CAD build for the part. Positions are in the model's coordinates, mm. A direction names the side the tool comes from. Give positions to 0.01 mm unless a question says otherwise; leave off trailing zeros. Write each loop counter-clockwise with the first axis right and the second up, starting at its lowest first coordinate (ties: lowest second). Pieces come first, ordered by that corner, then holes. Notation, with made-up numbers: M 48,37.25 L 81,37.25 A23 ccw 81,58.25 Z; hole C 31.25,49.25 d3. An arc over 180 degrees is marked long. One line per question, with ' | ' between items. Start each with the question number.
1. Cut at D-D, the plane x = 46.5. Write the cut outline in (y, z).
2. Wall check: L1, parallel to Y at x = -17.67, z = 1.6; L2, parallel to X at y = 0.75, z = 1.4; L3, parallel to X at y = -4, z = 0.7. Give the ranges that are in metal, low to high.
3. Cut at A-A, the plane y = 0. Write the cut outline in (x, z), then the cut area to 3 significant figures.
4. Pull direction Y, two halves, no side cores. Call faces 3 (the face through (18, 1, 0)), 4 (the face through (50.036, -2.721, 0.986)), 5 (the face through (-19.42, 0.08, 0.99)), 6 (the face through (1.617, -0.67, 0.986)): released by +Y, released by -Y, zero draft, split by the parting line, or undercut.
5. Cut at C-C, the plane z = 1.1. Write the cut outline in (x, y) (3 decimals), then the cut area to 3 significant figures.
6. Which spindle directions (+Z, -Z, +X, -X, +Y, -Y) get a long thin tool onto all of the face, cutting with end or side? Do faces 1 (the face through (-14.26, 4.01, 0.99)), 2 (the face through (-10, -3.125, 1)). Say none if no direction does.
7. Cut at B-B, the plane x = -17.67. Write the cut outline in (y, z), then the cut area to 3 significant figures.
```python
from build123d import *

# Parameters (mm, degrees)
SKETCH1_R           = 1.75
BOSS_EXTRUDE1_DEPTH = 2


with BuildPart() as part:
    # Sketch1 → Boss-Extrude1 (new body)
    with BuildSketch(Plane.XY):
        with BuildLine():
            Line((-1.959177489, 6.07006951), (-12.067534954, 4.175209114))
            ThreePointArc((-12.067534954, 4.175209114), (-14.294918054, 4.01142257), (-16.503100774, 4.346072502))
            ThreePointArc((-16.503100774, 4.346072502), (-22.152448054, -0.397063522), (-15.757299357, -4.073275862))
            ThreePointArc((-15.757299357, -4.073275862), (-13.684324334, -3.364947711), (-11.506853482, -3.125))
            Line((-11.506853482, -3.125), (-7.49859406, -3.125))
            ThreePointArc((-7.49859406, -3.125), (-5.373977874, -3.353305875), (-3.34637416, -4.027798787))
            ThreePointArc((-3.34637416, -4.027798787), (0, -4.75), (3.341869686, -4.007233812))
            ThreePointArc((3.341869686, -4.007233812), (5.310275247, -3.332763669), (7.375648406, -3.080248053))
            Line((7.375648406, -3.080248053), (47.281791607, -2.38455359))
            ThreePointArc((47.281791607, -2.38455359), (50.073909506, -2.731761792), (52.658788971, -3.843010658))
            ThreePointArc((52.658788971, -3.843010658), (59.498304049, -0.123534147), (52.873235099, 3.965711923))
            ThreePointArc((52.873235099, 3.965711923), (50.227695467, 2.997245413), (47.417022258, 2.8050907))
            Line((47.417022258, 2.8050907), (0.741973806, 6.221807217))
            ThreePointArc((0.741973806, 6.221807217), (-0.613509345, 6.233299043), (-1.959177489, 6.07006951))
        make_face()
        with Locations((-17.67, 0)):
            Circle(SKETCH1_R, mode=Mode.SUBTRACT)
        Circle(SKETCH1_R, mode=Mode.SUBTRACT)
        with Locations((55, 0)):
            Circle(SKETCH1_R, mode=Mode.SUBTRACT)
    extrude(amount=BOSS_EXTRUDE1_DEPTH)


solid = part.part
```
Here are the results:
1) outline: M -2.4,0 L 2.87,0 L 2.87,2 L -2.4,2 Z
2) L1: -4.5 to -1.75, 1.75 to 4.5 | L2: -22.11 to -19.25, -16.09 to -1.58, 1.58 to 53.42, 56.58 to 59.44 | L3: -19.73 to -15.6, -3.41 to 3.36, 52.94 to 57.06
3) outline: M -22.17,0 L -19.42,0 L -19.42,2 L -22.17,2 Z; M -15.92,0 L -1.75,0 L -1.75,2 L -15.92,2 Z; M 1.75,0 L 53.25,0 L 53.25,2 L 1.75,2 Z; M 56.75,0 L 59.5,0 L 59.5,2 L 56.75,2 Z | area: 142 mm^2
4) face 3: zero draft | face 4: released by -Y | face 5: undercut | face 6: undercut
5) outline: M -16.503,4.346 A4.5 ccw long -15.757,-4.073 A10 cw -11.507,-3.125 L -7.499,-3.125 A10 cw -3.346,-4.028 A8 ccw 3.342,-4.007 A10 cw 7.376,-3.08 L 47.282,-2.385 A10 cw 52.659,-3.843 A4.5 ccw long 52.873,3.966 A10 cw 47.417,2.805 L 0.742,6.222 A10.5 ccw -1.959,6.07 L -12.068,4.175 A10 cw Z; hole C -17.67,0 d3.5; hole C 0,0 d3.5; hole C 55,0 d3.5 | area: 591 mm^2
6) face 1: +Z, -Z, +Y | face 2: +Z, -Z, -Y
7) outline: M -4.5,0 L -1.75,0 L -1.75,2 L -4.5,2 Z; M 1.75,0 L 4.5,0 L 4.5,2 L 1.75,2 Z | area: 11.0 mm^2
